Check sheet for the modelled part. Datum: model origin and axes. Units: mm. Coordinates: 2 decimals unless noted, no trailing zeros. Order: outer loops, then holes, each group sorted by start corner. A loop starts at its lowest first (then second) coordinate and runs counter-clockwise, first axis right, second up.
from build123d import *

# Parameters (mm, degrees)
F0_R          = 4
F0_R_2        = 3.5
F1_DEPTH      = 330
F2_R          = 0.5
F3_DEPTH      = 4.001
F3_DEPTH_BACK = 25


with BuildPart() as f1:
    # F0 (on Top) → F1 (new body)
    with BuildSketch(Plane.XY):
        Circle(F0_R)
        Circle(F0_R_2, mode=Mode.SUBTRACT)
    extrude(amount=F1_DEPTH)

    # F2 (on Front) → F3 (cut, two sides)
    with BuildSketch(Plane.XZ) as f3_sk:
        with Locations((0, 5)):
            Circle(F2_R)
        with Locations((0, 305)):
            Circle(F2_R)
    extrude(amount=-F3_DEPTH, mode=Mode.SUBTRACT)
    extrude(f3_sk.sketch, amount=F3_DEPTH_BACK, mode=Mode.SUBTRACT)


solid = f1.part
(1) Go/stop test with flat-tipped pins: P1, Ø3, axis at x = 1.5, z = 49, coming from the +Y side; P2, Ø2, axis at y = 2, z = 142.5, coming from the -X side; P3, Ø2, axis at x = -2.5, z = 288.5, coming from the +Y side; P4, Ø1.5, axis at y = 2, z = 228, coming from the +X side. Record where each tip stops, or that it passes through.
Filled in:
P1: stops at y = 4
P2: stops at x = -3.87
P3: stops at y = 3.71
P4: stops at x = 3.8
(2) Thickness scan on probe 1 along Z at (x, y) = (0, -3.75); probe 2 along Y at (x, z) = (-0.25, 177); probe 3 along Y at (x, z) = (2.75, 269.5). Record the ranges inside material, lowest first.
Filled in:
probe 1: z = 0 to 4.5, 5.5 to 304.5, 305.5 to 330
probe 2: y = -3.99 to -3.49, 3.49 to 3.99
probe 3: y = -2.9 to -2.17, 2.17 to 2.9
(3) Cross-section at B-B (z = 252). Enter the section's corners in (x, y), and give its area (3 significant figures).
Filled in:
outline: circle Ø8 at (0, 0); hole circle Ø7 at (0, 0)
area: 11.8 mm2
(4) Cross-section at A-A (y = 0). Enter the section's corners in (x, z), and give its area (3 significant figures).
Filled in:
outline: (-4, 0) - (-3.5, 0) - (-3.5, 330) - (-4, 330) - close; (3.5, 0) - (4, 0) - (4, 330) - (3.5, 330) - close
area: 330 mm2
